Can you work these out from the model? Positions are in its coordinate system, mm. A direction names the side the tool comes from. Round coordinates to 2 decimals unless told otherwise and drop trailing zeros. Order: outer loops, then holes, each group sorted by start corner. A loop starts at its lowest first (then second) coordinate and runs counter-clockwise, first axis right, second up. Notation, with made-up numbers: (-7.5, 30.25) -> (35.5, 30.25) arc R20 cw to (35.5, 42.25) -> close; hole circle Ø2 at (-32.5, -10.75). An arc over 180 degrees is marked (long way). One line per item, written item: value.
```python
from build123d import *

# Parameters (mm, degrees)
SKETCH1_R           = 127
SKETCH1_R_2         = 16.7894
BOSS_EXTRUDE1_DEPTH = 82.9564
FILLET1_R           = 15.24
CUT_EXTRUDE1_START  = -35.2044
SKETCH2_R           = 88.9
SKETCH2_R_2         = 16.7894
CUT_EXTRUDE1_DEPTH  = 35.2044


with BuildPart() as part:
    # Sketch1 → Boss-Extrude1 (new body)
    with BuildSketch(Plane(origin=(0, 0, 0), x_dir=(0, 0, -1), z_dir=(1, 0, 0))):
        Circle(SKETCH1_R)
        Circle(SKETCH1_R_2, mode=Mode.SUBTRACT)
    extrude(amount=BOSS_EXTRUDE1_DEPTH)

    # Fillet1
    fillet1_edges = [part.edges().sort_by_distance(p)[0] for p in [
        (0, 0, 127),
        (82.9564, 0, 127),
    ]]
    fillet(fillet1_edges, radius=FILLET1_R)

    # Sketch2 → Cut-Extrude1 (cut)
    with BuildSketch(Plane(origin=(82.9564, 0, 0), x_dir=(0, 0, -1), z_dir=(1, 0, 0)).offset(CUT_EXTRUDE1_START)):
        Circle(SKETCH2_R)
        Circle(SKETCH2_R_2, mode=Mode.SUBTRACT)
    cut_extrude1 = extrude(amount=CUT_EXTRUDE1_DEPTH, mode=Mode.SUBTRACT)

    # Mirror1: Cut-Extrude1 across plane
    add(cut_extrude1.mirror(Plane.ZY.offset(-41.4782)), mode=Mode.SUBTRACT)


solid = part.part
```
Q1. I want a section at A-A on y = 0. List the corners of the cut face in (x, z) for me.
Answers below:
outline: (0, -111.76) arc R15.24 ccw to (15.24, -127) -> (67.72, -127) arc R15.24 ccw to (82.96, -111.76) -> (82.96, -88.9) -> (47.75, -88.9) -> (47.75, -16.79) -> (35.2, -16.79) -> (35.2, -88.9) -> (0, -88.9) -> close; (0, 88.9) -> (35.2, 88.9) -> (35.2, 16.79) -> (47.75, 16.79) -> (47.75, 88.9) -> (82.96, 88.9) -> (82.96, 111.76) arc R15.24 ccw to (67.72, 127) -> (15.24, 127) arc R15.24 ccw to (0, 111.76) -> close
Q2. Will these pins go through, and if not, where does the flat tip stop? pin 1 Ø1.5 at (y, z) = (30, -46) entering from -X; pin 2 Ø1.5 at (x, z) = (63, 76.5) entering from +Y; pin 3 Ø1.5 at (y, z) = (54.5, 58.5) entering from +X.
Answers below:
pin 1: x = 35.2
pin 2: y = 101.94
pin 3: x = 47.75
Q3. I want a section at C-C on x = 40. List the corners of the cut face in (y, z) for me, plus the area to 3 significant figures.
Answers below:
outline: circle Ø254 at (0, 0); hole circle Ø33.58 at (0, 0)
area: 49,800 mm^2
Q4. On a 3-axis mill with a long thin cutter (end or side, diameter ignored), from which of +Z, -Z, +X, -X, +Y, -Y can I reach the whole of each face in a straight line? I mean faces 1 (the face through (47.752, -19, 1)), 2 (the face through (82.956, -49, 75)), 3 (the face through (35.204, -19, 1)). Say none if no direction works.
Answers below:
face 1: +X
face 2: +Z, -Z, +X, +Y, -Y
face 3: -X
Q5. We'd pull the mould along Z, two halves only. Please class faces 4 (the face through (41.39, 5.043, -16.014)), 5 (the face through (0, -49, 75)), 6 (the face through (41.11, -123.98, 27.53)): released by +Z, released by -Z, zero draft, split by the parting line, or undercut.
Answers below:
face 4: undercut
face 5: zero draft
face 6: split by the parting line
Q6. Please list where these lines run through material, in increasing order: line 1 along Y through (x, z) = (55, 0); line 2 along Y through (x, z) = (39, 0); line 3 along X through (y, z) = (21.5, 76.5).
Answers below:
line 1: -127 to -88.9, 88.9 to 127
line 2: -127 to -16.79, 16.79 to 127
line 3: 35.2 to 47.75
Q7. I want a section at D-D on x = 18.5. List the corners of the cut face in (y, z) for me.
Answers below:
outline: circle Ø254 at (0, 0); hole circle Ø177.8 at (0, 0)
